Geometry: final body of the model. Coordinates: model frame, mm. A direction names the side the tool comes from. Give positions to 0.01 mm unless a question says otherwise; leave off trailing zeros. Write each loop counter-clockwise with the first axis right and the second up, starting at its lowest first coordinate (ties: lowest second). Pieces come first, ordered by that corner, then holes.
Q1. Cut plane C-C on x = 2.75. Return the cut outline in (y, z) (3 decimals), plus the area to 3 significant figures.
Q2. Cut plane D-D on z = -1.5. Return the cut outline in (x, y) (3 decimals), plus the area to 3 significant figures.
Q3. Pin query (flat end, axial travel): pin 1 (8 mm diameter, centred on x = 22.5, y = 14.5, fed in from -Z) (3 decimals); pin 2 (5.5 mm diameter, centred on x = 12.7, z = -12.7, fed in from +Y); pin 3 (6.5 mm diameter, centred on x = 17, z = -18.5, fed in from +Y) (3 decimals); pin 4 (1 mm diameter, centred on y = 17.5, z = -22, fed in from +X) (3 decimals). Return the tip coordinate at first contact, or that it passes through.
Q4. Line query: L1, parallel to Y at x = 12.7, z = -1.45 (3 decimals); L2, parallel to Z at x = 12.7, y = 2.25 (3 decimals); L3, parallel to X at y = 3.5, z = -13.25 (3 decimals). Output: solid intervals per line, ascending.
Q5. Reachability of faces 4 (the face through (2, 8, -25.4)), 5 (the face through (17, 14, -3.175)) from +Z, -Z, +X, -X, +Y, -Y: full face, straight path, thin tool, end or side. Return the list, or none.
Q6. Draft query along Z for faces 1 (the face through (1.6, 9.9, -11.2)), 2 (the face through (25.4, 7, -2)), 3 (the face through (15.3, 15.3, 0)). Return one class per face: pulls with the +Z half, pulls with the -Z half, needs draft (parallel to the pull), parting line crosses it, or undercut.
Q7. Cut plane A-A on x = 12.7. Return the cut outline in (y, z) (3 decimals).
Q8. Cut plane B-B on z = -12.7. Return the cut outline in (x, y) (3 decimals).
Autodesk Inventor part; units mm, degrees
ref_plane "YZ Plane" through (0, 0, 0) normal (1, 0, 0) x (0, 1, 0)
ref_plane "XZ Plane" through (0, 0, 0) normal (0, 1, 0) x (-1, 0, 0)
ref_plane "XY Plane" through (0, 0, 0) normal (0, 0, 1) x (1, 0, 0)
sketch "Sketch1" plane through (0, 0, 0) normal (0, 1, 0) x (-1, 0, 0)
  line L0 (0, 0) -> (-25.4, 0)
  line L1 (-25.4, 0) -> (-25.4, -25.4)
  line L2 (-25.4, -25.4) -> (0, -25.4)
  line L3 (0, -25.4) -> (0, 0)
  line L4 (0, 0) -> (-25.4, -25.4) construction
  line L5 (0, -25.4) -> (-25.4, 0) construction
  circle A0 centre (-12.7, -12.7) radius 3.175
  dimension "d0" = 25.4
  dimension "d1" = 25.4
  dimension "d2" = 6.35
extrude "Extrusion1" add sketch "Sketch1" along normal blind 3.175
sketch "Sketch2" plane through (0, 0, 0) normal (0, 0, 1) x (1, 0, 0)
  line L0 (0, 0) -> (0, 3.175)
  line L1 (0, 0) -> (25.4, 0)
  line L2 (25.4, 0) -> (25.4, 25.4)
  line L3 (25.4, 25.4) -> (0, 25.4)
  line L4 (0, 25.4) -> (0, 0)
  line L5 (25.4, 0) -> (25.4, 3.175) construction
  line L6 (0, 25.4) -> (25.4, 0) construction
  line L7 (25.4, 25.4) -> (0, 0) construction
  circle A0 centre (12.7, 12.7) radius 3.175
  dimension "d5" = 25.4
  dimension "d6" = 25.4
  dimension "d7" = 6.35
extrude "Extrusion2" add sketch "Sketch2" against normal blind 3.175
sketch "Sketch3" plane through (0, 0, -25.4) normal (-1, 0, 0) x (0, 0, 1)
  line L0 (0, 0) -> (25.4, 0)
  line L1 (25.4, 0) -> (25.4, 25.4)
  line L2 (0, 0) -> (25.4, 0)
  line L3 (25.4, 0) -> (25.4, 25.4)
  line L4 (25.4, 25.4) -> (0, 25.4)
  line L5 (0, 25.4) -> (0, 0)
  line L6 (0, 25.4) -> (25.4, 0) construction
  line L7 (25.4, 25.4) -> (0, 0) construction
  circle A0 centre (12.7, 12.7) radius 3.175
  dimension "d10" = 25.4
  dimension "d11" = 6.35
extrude "Extrusion3" add sketch "Sketch3" against normal blind 3.175
properties part number "MountingBracket"
Data:
1. outline: (0, -25.4) - (25.4, -25.4) - (25.4, 0) - (0, 0) - close; hole circle Ø6.35 at (12.7, -12.7)
1. area: 613 mm2
2. outline: (0, 0) - (25.4, 0) - (25.4, 25.4) - (0, 25.4) - close; hole circle Ø6.35 at (12.7, 12.7)
2. area: 613 mm2
3. pin 1: stops at z = -3.175
3. pin 2: passes through
3. pin 3: stops at y = 3.175
3. pin 4: stops at x = 3.175
4. L1: y = 0 to 9.525, 15.875 to 25.4
4. L2: z = -25.4 to -15.875, -9.525 to 0
4. L3: x = 0 to 3.175
5. face 4: -Z, +X, -X, +Y, -Y
5. face 5: -Z, +X, +Y
6. face 1: undercut
6. face 2: needs draft
6. face 3: pulls with the +Z half
7. outline: (0, -25.4) - (3.175, -25.4) - (3.175, -15.875) - (0, -15.875) - close; (0, -9.525) - (3.175, -9.525) - (3.175, -3.175) - (9.525, -3.175) - (9.525, 0) - (0, 0) - close; (15.875, -3.175) - (25.4, -3.175) - (25.4, 0) - (15.875, 0) - close
8. outline: (0, 0) - (9.525, 0) - (9.525, 3.175) - (3.175, 3.175) - (3.175, 9.525) - (0, 9.525) - close; (0, 15.875) - (3.175, 15.875) - (3.175, 25.4) - (0, 25.4) - close; (15.875, 0) - (25.4, 0) - (25.4, 3.175) - (15.875, 3.175) - close
